Can you work these out from the drawing? Everything is in mm from the part's minimum corner. Round coordinates to 2 decimals unless told otherwise and drop trailing zeros. Order: outer loops, then holes, each group sorted by start corner. A loop starts at its lowest first (then second) coordinate and runs counter-clockwise, first axis right, second up. Notation, with made-up numbers: (85.5, -21.75) - (102.5, -21.75) arc R8 cw to (102.5, -6.75) - close; hole circle Ø4 at (9, 64). An arc over 180 degrees is marked (long way). Answer as a JSON object with one key per item and string values.
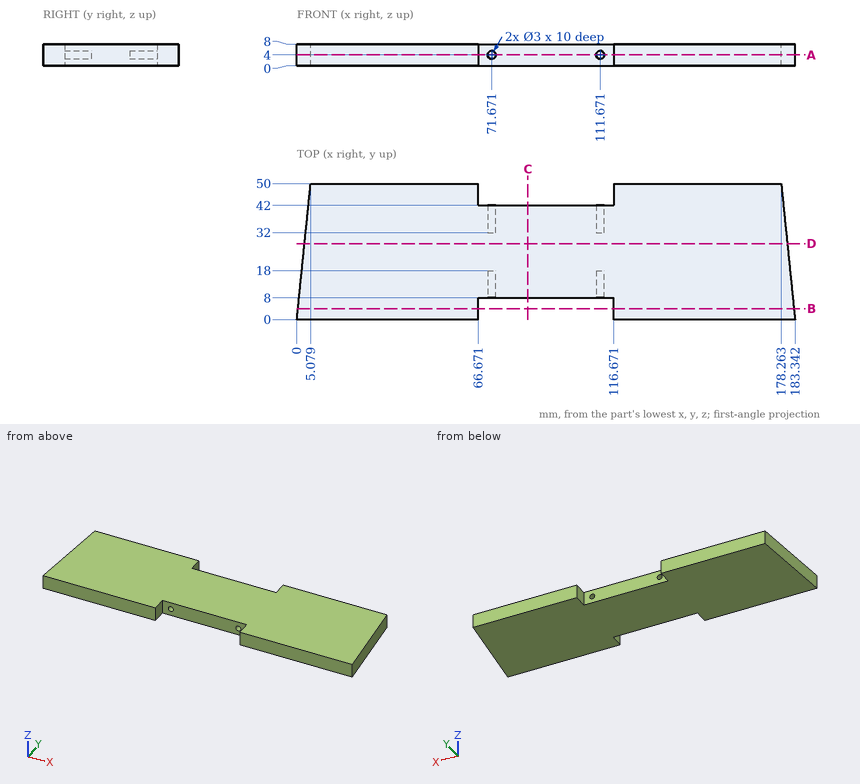
1. If I drill on L1, parallel to X at y = 14.5, z = 4; L2, parallel to X at y = 37, z = 3; L3, parallel to X at y = 43.5, z = 5.5, over which ranges is the centre line in solid material (lowest first)? Write a range as [from, to].
Responses:
{"L1": "[1.47, 70.17], [73.17, 110.17], [113.17, 181.87]", "L2": "[3.76, 70.55], [72.79, 110.55], [112.79, 179.58]", "L3": "[4.42, 66.67], [116.67, 178.92]"}
2. Imagine slicing it at A-A (z = 4). List the corners of the cut face in (x, y) for me.
Responses:
{"outline": "(0, 0) - (66.67, 0) - (66.67, 8) - (70.17, 8) - (70.17, 18) - (73.17, 18) - (73.17, 8) - (110.17, 8) - (110.17, 18) - (113.17, 18) - (113.17, 8) - (116.67, 8) - (116.67, 0) - (183.34, 0) - (178.26, 50) - (116.67, 50) - (116.67, 42) - (113.17, 42) - (113.17, 32) - (110.17, 32) - (110.17, 42) - (73.17, 42) - (73.17, 32) - (70.17, 32) - (70.17, 42) - (66.67, 42) - (66.67, 50) - (5.08, 50) - close"}
3. Imagine slicing it at B-B (y = 4). List the corners of the cut face in (x, z) for me (1 decimal).
Responses:
{"outline": "(0.4, 0) - (66.7, 0) - (66.7, 8) - (0.4, 8) - close; (116.7, 0) - (182.9, 0) - (182.9, 8) - (116.7, 8) - close"}
4. Imagine slicing it at C-C (x = 85). List the corners of the cut face in (y, z) for me, plus the area to 3 significant figures.
Responses:
{"outline": "(8, 0) - (42, 0) - (42, 8) - (8, 8) - close", "area": "272 mm2"}
5. Imagine slicing it at D-D (y = 28). List the corners of the cut face in (x, z) for me.
Responses:
{"outline": "(2.84, 0) - (180.5, 0) - (180.5, 8) - (2.84, 8) - close"}
6. For P1, Ø2.5, axis at y = 47.5, z = 5, coming from the -X side; P2, Ø4, axis at x = 71.67, z = 4, coming from the +Y side; P3, Ø3.5, axis at x = 71.5, z = 4, coming from the -Y side, each with a flat end and sliding along its axis, tell me the tip position at first contact or that it passes through.
Responses:
{"P1": "x = 4.7", "P2": "y = 42", "P3": "y = 8"}
